```python
from build123d import *

# Parameters (mm, degrees)
SKETCH1_W           = 25.4
SKETCH1_H           = 25.4
BOSS_EXTRUDE1_DEPTH = 25.4
SHELL1_T            = -2
SKETCH2_R           = 0.5
CUT_EXTRUDE1_DEPTH  = 6.4
SKETCH3_R           = 0.5
CUT_EXTRUDE2_DEPTH  = 6.4
SKETCH5_W           = 24
SKETCH5_H           = 24
CUT_EXTRUDE3_DEPTH  = 1.5


with BuildPart() as part:
    # Sketch1 → Boss-Extrude1 (new body)
    with BuildSketch(Plane(origin=(0, 0, 0), x_dir=(1, 0, 0), z_dir=(0, 1, 0))):
        Rectangle(SKETCH1_W, SKETCH1_H)
    extrude(amount=BOSS_EXTRUDE1_DEPTH)

    # Shell1
    shell1_openings = [part.faces().sort_by_distance(p)[0] for p in [
        (0, 25.4, 0),
    ]]
    offset(amount=SHELL1_T, openings=shell1_openings, kind=Kind.INTERSECTION)

    # Sketch2 → Cut-Extrude1 (cut)
    with BuildSketch(Plane(origin=(12.7, 0, 0), x_dir=(0, 0, -1), z_dir=(1, 0, 0))):
        with Locations((0, 10.5)):
            Circle(SKETCH2_R)
    extrude(amount=-CUT_EXTRUDE1_DEPTH, mode=Mode.SUBTRACT)

    # Sketch3 → Cut-Extrude2 (cut)
    with BuildSketch(Plane(origin=(12.7, 0, 0), x_dir=(0, 0, -1), z_dir=(1, 0, 0))):
        with Locations((0, 14.9)):
            Circle(SKETCH3_R)
    extrude(amount=-CUT_EXTRUDE2_DEPTH, mode=Mode.SUBTRACT)

    # Sketch5 → Cut-Extrude3 (cut)
    with BuildSketch(Plane.ZY.offset(12.7)):
        with Locations((0, 12.7)):
            Rectangle(SKETCH5_W, SKETCH5_H)
    extrude(amount=-CUT_EXTRUDE3_DEPTH, mode=Mode.SUBTRACT)


solid = part.part
```
Could you check a few things on this model? Use its own coordinates, in mm. A direction names the side the tool comes from. Round coordinates to 2 decimals unless told otherwise and drop trailing zeros. Write each loop counter-clockwise with the first axis right and the second up, starting at its lowest first coordinate (ties: lowest second). Pieces come first, ordered by that corner, then holes. Notation, with made-up numbers: M 10.5,-2 L 25.5,-2 A24 ccw 25.5,28 Z; hole C -7,74 d3. An arc over 180 degrees is marked long. Answer in a Markdown table with one row per item. Add a question column.
Q1. Imagine slicing it at B-B (y = 14.9). Please give me the cut outline in (x, z).
Q2. On a 3-axis mill with a long thin cutter (end or side, diameter ignored), from which of +Z, -Z, +X, -X, +Y, -Y can I reach the whole of each face in a straight line? I mean faces 1 (the flat face through (12.7, 13, 0)), 2 (the flat face through (-12.7, 25, 1)), 3 (the cylindrical face through (11.714, 14.412, 0.108)), 4 (the flat face through (-10.7, 14, 0)), 5 (the flat face through (-12, 13, 12)). Say none if no direction works.
Q3. If we mould it in two halves opening along Y, with no side actions, what happens to faces 6 (the flat face through (0, 14, 10.7)), 7 (the flat face through (-12, 0.7, 0)), 8 (the flat face through (11, 25.4, 0)), 9 (the flat face through (0, 0, 0))? For each: +Y half, -Y half, draft (parallel to the pull), parting line (faces both ways), or undercut.
Q4. Imagine slicing it at D-D (y = 20.5). Please give me the cut outline in (x, z), then the cut area to 3 significant figures.
Q5. Will these pins go through, and if not, where does the flat tip stop? pin 1 Ø1.6 at (x, z) = (-12.5, 1) entering from -Y; pin 2 Ø3 at (y, z) = (3.5, -2.5) entering from -X; pin 3 Ø4 at (x, z) = (5, -1.5) entering from +Y.
Q6. Imagine slicing it at C-C (z = 4.75). Please give me the cut outline in (x, y).
Q7. If I drill on line 1 (Y direction, x = 12.15, z = 0); line 2 (X direction, y = 4.75, z = 2.25); line 3 (Z direction, x = 10, y = 24), over which ranges is the centre line in solid material (lowest first)? Write a range as from..to.
Q8. Imagine slicing it at A-A (x = 5.5). Please give me the cut outline in (y, z), then the cut area to 3 significant figures.
Values:
| question | item | result |
|---|---|---|
| 1 | outline | M -12.7,-12.7 L 12.7,-12.7 L 12.7,-0.5 L 10.7,-0.5 L 10.7,-10.7 L -10.7,-10.7 L -10.7,10.7 L 10.7,10.7 L 10.7,0.5 L 12.7,0.5 L 12.7,12.7 L -12.7,12.7 L -12.7,12 L -11.2,12 L -11.2,-12 L -12.7,-12 Z |
| 2 | face 1 | +Z, -Z, +X, +Y, -Y |
| 2 | face 2 | +Z, -Z, -X, +Y, -Y |
| 2 | face 3 | +X |
| 2 | face 4 | +Y |
| 2 | face 5 | -X |
| 3 | face 6 | draft |
| 3 | face 7 | undercut |
| 3 | face 8 | +Y half |
| 3 | face 9 | -Y half |
| 4 | outline | M -12.7,-12.7 L 12.7,-12.7 L 12.7,12.7 L -12.7,12.7 L -12.7,12 L -11.2,12 L -11.2,-12 L -12.7,-12 Z; hole M -10.7,-10.7 L 10.7,-10.7 L 10.7,10.7 L -10.7,10.7 Z |
| 4 | area | 151 mm^2 |
| 5 | pin 1 | y = 0 |
| 5 | pin 2 | x = -11.2 |
| 5 | pin 3 | y = 2 |
| 6 | outline | M -12.7,0 L 12.7,0 L 12.7,25.4 L 10.7,25.4 L 10.7,2 L -10.7,2 L -10.7,25.4 L -12.7,25.4 L -12.7,24.7 L -11.2,24.7 L -11.2,0.7 L -12.7,0.7 Z |
| 7 | line 1 | 0..10, 11..14.4, 15.4..25.4 |
| 7 | line 2 | -11.2..-10.7, 10.7..12.7 |
| 7 | line 3 | -12.7..-10.7, 10.7..12.7 |
| 8 | outline | M 0,-12.7 L 25.4,-12.7 L 25.4,-10.7 L 2,-10.7 L 2,10.7 L 25.4,10.7 L 25.4,12.7 L 0,12.7 Z |
| 8 | area | 144 mm^2 |
